from build123d import *

# Parameters (mm, degrees)
EXTRUDE_1_DEPTH     = 1
CHAMFER_1_SIZE      = 0.6
SKETCH_2_W          = 14.8
SKETCH_2_H          = 4
EXTRUDE_2_DEPTH     = 1
EXTRUDE_3_DEPTH     = 3
SKETCH_4_R          = 1.2
CUT_EXTRUDE_1_DEPTH = 78.515546828
SKETCH_5_R          = 2.05
CUT_EXTRUDE_2_DEPTH = 2
CHAMFER_2_SIZE      = 1


with BuildPart() as part:
    # 草图1 → 凸台-拉伸1 (new body)
    with BuildSketch(Plane(origin=(0, 0, 0), x_dir=(1, 0, 0), z_dir=(0, 1, 0))):
        Polygon((0, 0), (37.9, 0), (37.9, 62.5), (36.9, 63.5), (35.9, 63.5), (33.9, 65.5), (19.1, 65.5), (17.1, 63.5), (2.5, 63.5), (1.5, 62.5), (1.5, 21.5), (0, 20), align=None)
    extrude(amount=EXTRUDE_1_DEPTH)

    # 倒角1
    chamfer_1_edges = [part.edges().sort_by_distance(p)[0] for p in [
        (0.75, 0, -20.75),
        (1.5, 0, -42),
        (2, 0, -63),
        (9.8, 0, -63.5),
        (18.1, 0, -64.5),
        (26.5, 0, -65.5),
        (34.9, 0, -64.5),
        (36.4, 0, -63.5),
        (37.4, 0, -63),
        (37.9, 0, -31.25),
        (18.95, 0, 0),
        (0, 0, -10),
    ]]
    chamfer(chamfer_1_edges, length=CHAMFER_1_SIZE)

    # 草图2 → 凸台-拉伸2 (add)
    with BuildSketch(Plane(origin=(0, 1, 0), x_dir=(1, 0, 0), z_dir=(0, 1, 0))):
        with Locations((26.5, 65.5)):
            Rectangle(SKETCH_2_W, SKETCH_2_H)
    extrude(amount=EXTRUDE_2_DEPTH)

    # 草图3 → 凸台-拉伸3 (add)
    with BuildSketch(Plane(origin=(0, 1, 0), x_dir=(1, 0, 0), z_dir=(0, 1, 0))):
        with BuildLine():
            Line((5, 4), (5, 0))
            Line((5, 0), (11, 0))
            Line((11, 0), (11, 4))
            ThreePointArc((11, 4), (10.414213562, 5.414213562), (9, 6))
            Line((9, 6), (7, 6))
            ThreePointArc((7, 6), (5.585786438, 5.414213562), (5, 4))
        make_face()
    extrude(amount=EXTRUDE_3_DEPTH)

    # 草图4 → 切除-拉伸1 (cut, through all)
    with BuildSketch(Plane.XZ):
        with Locations(Location((8, -3.05, 0), (0, 0, 270))):
            Circle(SKETCH_4_R)
    extrude(amount=-CUT_EXTRUDE_1_DEPTH, mode=Mode.SUBTRACT)

    # 草图5 → 切除-拉伸2 (cut)
    with BuildSketch(Plane.XZ):
        with Locations(Location((8, -3.05, 0), (0, 0, 270))):
            Circle(SKETCH_5_R)
    extrude(amount=-CUT_EXTRUDE_2_DEPTH, mode=Mode.SUBTRACT)

    # 倒角2
    chamfer_2_edges = [part.edges().sort_by_distance(p)[0] for p in [
        (26.5, 2, -63.5),
    ]]
    chamfer(chamfer_2_edges, length=CHAMFER_2_SIZE - 0.0001)  # a hair under: the kernel refuses the full size


solid = part.part
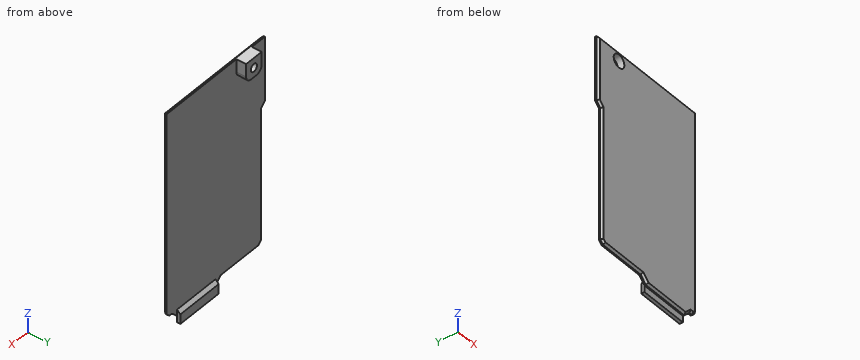
Input: part model. Units: mm. Frame: model coordinates. Round coordinates to 2 decimals unless told otherwise and drop trailing zeros. Order: outer loops, then holes, each group sorted by start corner. A loop starts at its lowest first (then second) coordinate and runs counter-clockwise, first axis right, second up. Notation, with made-up numbers: (-17.75, 86.25) - (32.25, 86.25) arc R11 ccw to (32.25, 101.25) - close; hole circle Ø9 at (36.25, 70.25). An arc over 180 degrees is marked (long way). Answer as a JSON object with one key per item and string values. Group by question number.
(1) Material intervals for probe 1 along X at (y, z) = (0.7, -3.05); probe 2 along Y at (x, z) = (11.5, -57.5); probe 3 along X at (y, z) = (1.05, -3), sorted ascending. Write a range as from..to.
(2) Pin query (flat end, axial travel): P1, Ø2.5, axis at x = 8, z = -3.05, coming from the +Y side; P2, Ø1, axis at x = 8, y = 2.5, coming from the -Z side; P3, Ø11.5, axis at x = 25, z = -18.5, coming from the +Y side; P4, Ø1.6, axis at x = 27.5, z = -66.5, coming from the -Y side. Return the tip coordinate at first contact, or that it passes through.
(3) Cut plane B-B (y = 3.3). Return loops of the section in (x, z).
(4) Cut plane C-C (z = -3.05). Return loops of the section in (x, y).
(5) Cut plane A-A (x = 8). Return loops of the section in (y, z), then the cut area to 3 significant figures.
Here are the results:
{
 "1": {"probe 1": "x = 0..5.95, 10.05..37.9", "probe 2": "y = 0..1", "probe 3": "x = 5..5.95, 10.05..11"},
 "2": {"P1": "stops at y = 4", "P2": "stops at z = -6", "P3": "stops at y = 1", "P4": "stops at y = 1"},
 "3": {"outline": "(5, -4) arc R2 ccw to (7, -6) - (9, -6) arc R2 ccw to (11, -4) - (11, 0) - (5, 0) - close; hole circle Ø2.4 at (8, -3.05)"},
 "4": {"outline": "(0, 0.6) - (0.6, 0) - (5.95, 0) - (5.95, 2) - (6.8, 2) - (6.8, 4) - (5, 4) - (5, 1) - (0, 1) - close; (9.2, 2) - (10.05, 2) - (10.05, 0) - (37.3, 0) - (37.9, 0.6) - (37.9, 1) - (11, 1) - (11, 4) - (9.2, 4) - close"},
 "5": {"outline": "(0, -62.9) - (0.6, -63.5) - (1, -63.5) - (1, -6) - (4, -6) - (4, -4.25) - (2, -4.25) - (2, -5.1) - (0, -5.1) - close; (0, -1) - (2, -1) - (2, -1.85) - (4, -1.85) - (4, 0) - (0.6, 0) - (0, -0.6) - close", "area": "68.1 mm^2"}
}
